For this review, take the finished solid that the model builds, in its own axes (mm). A direction names the side the tool comes from. Round coordinates to 2 decimals unless told otherwise and drop trailing zeros. Write each loop counter-clockwise with the first axis right and the second up, starting at its lowest first coordinate (ties: lowest second). Pieces come first, ordered by that corner, then holes. Notation, with made-up numbers: (85.25, 14) - (115.25, 14) arc R19 ccw to (115.25, 45) - close; hole circle Ø1 at (5, 88). An arc over 180 degrees is marked (long way). One line per item, written item: value. Start each with the question number.
Q1. Clearance check with flat-ended pins moving along their axes: pin 1 Ø1.5 at (y, z) = (14.5, 5) entering from +X; pin 2 Ø1 at (y, z) = (-11, 1) entering from -X; pin 3 Ø1.2 at (y, z) = (0, 7) entering from +X; pin 4 Ø1.9 at (x, y) = (13.5, 19) entering from +Z. State where each tip first meets the part, or that it passes through.
Q2. Add section B-B on y = -2. Write out the cut boundary in (x, z).
Q3. Mouldability with a two-part tool opening along X and no side actions: class faces 1 (the face through (-14.242, 0, 4)), 2 (the face through (10.893, -22.456, 3.944)), 3 (the face through (-0.14, -26.74, 3.94)), 4 (the face through (14.597, -14.854, 3.944)) as +X half, -X half, draft (parallel to the pull), parting line (faces both ways), or undercut.
Q4. For probe 1 along Y at (x, z) = (-13.5, 5); probe 2 along X at (y, z) = (-12.5, 0.7); probe 3 along X at (y, z) = (-4.5, 5), list the stretches that pass through material, from the lowest coordinate up.
Q5. Add section A-A on x = 0. Write out the cut boundary in (y, z).
Q6. Tool access review of faces 5 (the face through (14.576, 14.807, 3.944)), 6 (the face through (-9.7, -1.6, 8)), 7 (the face through (-0.22, 22.54, 7.26)): name each direction out of +Z, -Z, +X, -X, +Y, -Y from which nothing blocks a thin tool from reaching the whole face with its end or side.
Q7. Add section C-C on z = 1. Write out the cut boundary in (x, y), and give its area (3 significant figures).
Q8. Add section D-D on x = 13.5. Write out the cut boundary in (y, z).
```python
from build123d import *

# Parameters (mm, degrees)
SKETCH_1_R          = 6.25
EXTRUDE_1_DEPTH     = 8
CUT_EXTRUDE_START   = 2
CUT_EXTRUDE_1_DEPTH = 31.682534896
CUT_EXTRUDE_START_2 = 8
CUT_EXTRUDE_4_DEPTH = 1.5
HOLE_WIZARD_M3_2_D  = 3.2


with BuildPart() as part:
    # ｽｹｯﾁ1 → ﾎﾞｽ - 押し出し1 (new body)
    with BuildSketch(Plane.XY):
        with BuildLine():
            Line((-14.242252845, 12.5), (-14.242252845, -12.5))
            ThreePointArc((-14.242252845, -12.5), (-14.23978335, -12.765209825), (-14.232375721, -13.030327679))
            ThreePointArc((-14.232375721, -13.030327679), (-14.58644356, -14.830756402), (-15.707147454, -16.28366053))
            ThreePointArc((-15.707147454, -16.28366053), (-16.653505844, -20.518354666), (-12.752931254, -22.419340329))
            ThreePointArc((-12.752931254, -22.419340329), (-10.918262125, -22.449287076), (-9.290000484, -23.295260864))
            ThreePointArc((-9.290000484, -23.295260864), (0, -26.742252845), (9.290000484, -23.295260864))
            ThreePointArc((9.290000484, -23.295260864), (10.918262125, -22.449287076), (12.752931254, -22.419340329))
            ThreePointArc((12.752931254, -22.419340329), (16.653505844, -20.518354666), (15.707147454, -16.28366053))
            ThreePointArc((15.707147454, -16.28366053), (14.58644356, -14.830756402), (14.232375721, -13.030327679))
            ThreePointArc((14.232375721, -13.030327679), (14.23978335, -12.765209825), (14.242252845, -12.5))
            Line((14.242252845, -12.5), (14.242252845, 12.5))
            ThreePointArc((14.242252845, 12.5), (14.23978335, 12.765209825), (14.232375721, 13.030327679))
            ThreePointArc((14.232375721, 13.030327679), (14.58644356, 14.830756402), (15.707147454, 16.28366053))
            ThreePointArc((15.707147454, 16.28366053), (16.653505844, 20.518354666), (12.752931254, 22.419340329))
            ThreePointArc((12.752931254, 22.419340329), (10.918262125, 22.449287076), (9.290000484, 23.295260864))
            ThreePointArc((9.290000484, 23.295260864), (0, 26.742252845), (-9.290000484, 23.295260864))
            ThreePointArc((-9.290000484, 23.295260864), (-10.918262125, 22.449287076), (-12.752931254, 22.419340329))
            ThreePointArc((-12.752931254, 22.419340329), (-16.653505844, 20.518354666), (-15.707147454, 16.28366053))
            ThreePointArc((-15.707147454, 16.28366053), (-14.58644356, 14.830756402), (-14.232375721, 13.030327679))
            ThreePointArc((-14.232375721, 13.030327679), (-14.23978335, 12.765209825), (-14.242252845, 12.5))
        make_face()
        with Locations((0, 12.5)):
            Circle(SKETCH_1_R, mode=Mode.SUBTRACT)
        with Locations(Location((0, -12.5, 0), (0, 0, 180))):
            Circle(SKETCH_1_R, mode=Mode.SUBTRACT)
    extrude(amount=EXTRUDE_1_DEPTH)

    # ｽｹｯﾁ1<3> → ｶｯﾄ - 押し出し1 (cut, through all)
    with BuildSketch(Plane.XY.offset(CUT_EXTRUDE_START)):
        with BuildLine():
            Line((-9, 12.5), (-9, -12.5))
            ThreePointArc((-9, -12.5), (0, -21.5), (9, -12.5))
            Line((9, -12.5), (9, 12.5))
            ThreePointArc((9, 12.5), (0, 21.5), (-9, 12.5))
        make_face()
    extrude(amount=CUT_EXTRUDE_1_DEPTH, mode=Mode.SUBTRACT)

    # ｽｹｯﾁ1<6> → ｶｯﾄ - 押し出し4 (cut)
    with BuildSketch(Plane.XY.offset(CUT_EXTRUDE_START_2)):
        with BuildLine():
            ThreePointArc((12.742252845, -12.5), (0, -25.242252845), (-12.742252845, -12.5))
            Line((-12.742252845, -12.5), (-12.742252845, 12.5))
            ThreePointArc((-12.742252845, 12.5), (0, 25.242252845), (12.742252845, 12.5))
            Line((12.742252845, 12.5), (12.742252845, -12.5))
        make_face()
        with BuildLine():
            Line((10.042252845, 12.5), (10.042252845, -12.5))
            ThreePointArc((10.042252845, -12.5), (0, -22.542252845), (-10.042252845, -12.5))
            Line((-10.042252845, -12.5), (-10.042252845, 12.5))
            ThreePointArc((-10.042252845, 12.5), (0, 22.542252845), (10.042252845, 12.5))
        make_face(mode=Mode.SUBTRACT)
    extrude(amount=-CUT_EXTRUDE_4_DEPTH, mode=Mode.SUBTRACT)

    # M3 すきま穴2 (through all)
    with Locations(Plane(origin=(-13.5, 19, 0), x_dir=(-1, 0, 0), z_dir=(0, 0, -1))):
        with Locations((0, 0), (0, -38), (-27, -38), (-27, 0)):
            Hole(HOLE_WIZARD_M3_2_D / 2)


solid = part.part
```
Result set:
1. pin 1: stops at x = 14.81
1. pin 2: stops at x = -14.24
1. pin 3: stops at x = 14.24
1. pin 4: passes through
2. outline: (-14.24, 0) - (14.24, 0) - (14.24, 8) - (12.74, 8) - (12.74, 6.5) - (10.04, 6.5) - (10.04, 8) - (9, 8) - (9, 2) - (-9, 2) - (-9, 8) - (-10.04, 8) - (-10.04, 6.5) - (-12.74, 6.5) - (-12.74, 8) - (-14.24, 8) - close
3. face 1: -X half
3. face 2: undercut
3. face 3: parting line
3. face 4: +X half
4. probe 1: y = -22.5 to -20.6, -17.4 to 17.4, 20.6 to 22.5
4. probe 2: x = -14.24 to -6.25, 6.25 to 14.24
4. probe 3: x = -14.24 to -9, 9 to 14.24
5. outline: (-26.74, 0) - (-18.75, 0) - (-18.75, 2) - (-21.5, 2) - (-21.5, 8) - (-22.54, 8) - (-22.54, 6.5) - (-25.24, 6.5) - (-25.24, 8) - (-26.74, 8) - close; (-6.25, 0) - (6.25, 0) - (6.25, 2) - (-6.25, 2) - close; (18.75, 0) - (26.74, 0) - (26.74, 8) - (25.24, 8) - (25.24, 6.5) - (22.54, 6.5) - (22.54, 8) - (21.5, 8) - (21.5, 2) - (18.75, 2) - close
6. face 5: +Z, -Z, +X
6. face 6: +Z, +X, -X, +Y, -Y
6. face 7: +Z
7. outline: (-15.71, -16.28) arc R3.5 ccw to (-12.75, -22.42) arc R4 cw to (-9.29, -23.3) arc R14.24 ccw to (9.29, -23.3) arc R4 cw to (12.75, -22.42) arc R3.5 ccw to (15.71, -16.28) arc R4 cw to (14.23, -13.03) arc R14.24 ccw to (14.24, -12.5) - (14.24, 12.5) arc R14.24 ccw to (14.23, 13.03) arc R4 cw to (15.71, 16.28) arc R3.5 ccw to (12.75, 22.42) arc R4 cw to (9.29, 23.3) arc R14.24 ccw to (-9.29, 23.3) arc R4 cw to (-12.75, 22.42) arc R3.5 ccw to (-15.71, 16.28) arc R4 cw to (-14.23, 13.03) arc R14.24 ccw to (-14.24, 12.5) - (-14.24, -12.5) arc R14.24 ccw to (-14.23, -13.03) arc R4 cw to start; hole circle Ø3.2 at (-13.5, -19); hole circle Ø3.2 at (-13.5, 19); hole circle Ø12.5 at (0, -12.5); hole circle Ø12.5 at (0, 12.5); hole circle Ø3.2 at (13.5, -19); hole circle Ø3.2 at (13.5, 19)
7. area: 1,180 mm^2
8. outline: (-22.5, 0) - (-20.6, 0) - (-20.6, 8) - (-22.5, 8) - close; (-17.4, 0) - (17.4, 0) - (17.4, 8) - (-17.4, 8) - close; (20.6, 0) - (22.5, 0) - (22.5, 8) - (20.6, 8) - close
